Source: CAD feature listing. Evaluate the final solid. Frame: model axes, mm. Face numbers are marked on the shaded views. A direction names the side the tool comes from. Coordinates: 2 decimals unless noted, no trailing zeros. Write each loop counter-clockwise with the first axis right and the second up, starting at its lowest first coordinate (ties: lowest second). Pieces come first, ordered by that corner, then holes. Notation, with made-up numbers: (71, 26.25) -> (80, 26.25) arc R15 cw to (80, 41.25) -> close; hole circle Ø11 at (-2, 32.5). An arc over 180 degrees is marked (long way). One line per item, written item: value. Start each with the question number.
1. Section query A-A, the plane z = -31. Output: boundary loops of the cut face in (x, y), and give its area (3 significant figures).
2. Access query for the marked faces 4, 5, 6 and 7. Directions: +Z, -Z, +X, -X, +Y, -Y. A direction counts if a zero-diameter tool reaches every point of the face in a straight line with its end or side. Return the directions, or none.
3. Line query: line 1 (Y direction, x = -26, z = -4); line 2 (Z direction, x = -19.5, y = -22); line 3 (X direction, y = -29.5, z = -47). Output: solid intervals per line, ascending.
4. First-contact query: P1, Ø6, axis at x = 5, z = 36.5, coming from the +Y side; P2, Ø6, axis at x = 6, z = 11.5, coming from the -Y side; P3, Ø21.5, axis at y = 32.5, z = 18, coming from the -X side. Flat tips, straight axial feed; report the tip coordinate or a pass-through.
5. Mould query, pull axis Z, two halves, no side actions, for the marked faces 1, 2 and 3. Classes: released by +Z, released by -Z, zero draft, split by the parting line, or undercut.
from build123d import *

# Parameters (mm, degrees)
ENL_V_MAT_EXTRU_1_DEPTH      = 93.748315349
ENL_V_MAT_EXTRU_1_DEPTH_BACK = 93.748315349
ESQUISSE3_W                  = 49.590285902
ESQUISSE3_H                  = 55.327856271
ENL_V_MAT_EXTRU_2_DEPTH      = 93.748315349
ENL_V_MAT_EXTRU_2_DEPTH_BACK = 93.748315349


with BuildPart() as part:
    # Esquisse1 → Révolution1 (revolve)
    with BuildSketch(Plane(origin=(0, 0, 0), x_dir=(0, 0, -1), z_dir=(1, 0, 0)), mode=Mode.PRIVATE) as r_volution1_sk:
        with BuildLine():
            Line((-73.5, 0), (73.5, 0))
            Line((73.5, 0), (73.5, 25))
            Line((73.5, 25), (54.5, 25))
            ThreePointArc((54.5, 25), (53.085786438, 25.585786438), (52.5, 27))
            Line((52.5, 27), (52.5, 40))
            Line((52.5, 40), (21, 40))
            Line((21, 40), (18.5, 37.5))
            Line((18.5, 37.5), (-18.5, 37.5))
            Line((-18.5, 37.5), (-21, 40))
            Line((-21, 40), (-52.5, 40))
            Line((-52.5, 40), (-52.5, 27))
            ThreePointArc((-52.5, 27), (-53.085786438, 25.585786438), (-54.5, 25))
            Line((-54.5, 25), (-73.5, 25))
            Line((-73.5, 25), (-73.5, 0))
        make_face()
    revolve(r_volution1_sk.sketch.rotate(Axis((0, 0, 73.5), (0, 0, -1)), 90), axis=Axis((0, 0, 73.5), (0, 0, -1)))

    # Esquisse3 → Enlèv. mat.-Extru.1 (cut, two sides: drawn at the far end of the back side and taken through both)
    with BuildSketch(Plane.XY.offset(-ENL_V_MAT_EXTRU_1_DEPTH_BACK)):
        with Locations((-24.795142951, 27.663928136)):
            Rectangle(ESQUISSE3_W, ESQUISSE3_H)
    extrude(amount=ENL_V_MAT_EXTRU_1_DEPTH + ENL_V_MAT_EXTRU_1_DEPTH_BACK, mode=Mode.SUBTRACT)

    # Esquisse4 → Enlèv. mat.-Extru.2 (cut, two sides: drawn at the far end of the back side and taken through both)
    with BuildSketch(Plane.XY.offset(-ENL_V_MAT_EXTRU_2_DEPTH_BACK)):
        with BuildLine():
            Line((0, 7), (12, 7))
            ThreePointArc((12, 7), (15, 10), (12, 13))
            Line((12, 13), (0, 13))
            Line((0, 13), (0, 7))
        make_face()
    extrude(amount=ENL_V_MAT_EXTRU_2_DEPTH + ENL_V_MAT_EXTRU_2_DEPTH_BACK, mode=Mode.SUBTRACT)


solid = part.part
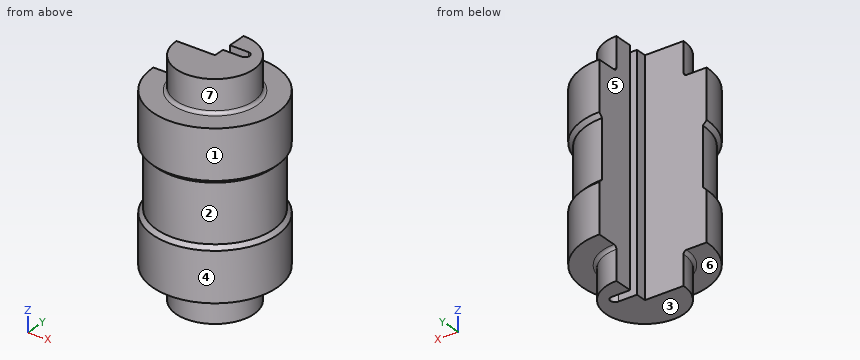
Computed values:
1. outline: (-40, 0) arc R40 ccw (long way) to (0, 40) -> (0, 13) -> (12, 13) arc R3 cw to (12, 7) -> (0, 7) -> (0, 0) -> close
1. area: 3,680 mm²
2. face 4: +Z, -Z
2. face 5: +Z, -Z, -X, +Y
2. face 6: -Z
2. face 7: +Z
3. line 1: y = -27.02 to 0
3. line 2: z = -52.5 to 52.5
3. line 3: x = -27.01 to 27.01
4. P1: stops at y = 39.95
4. P2: stops at y = -37.38
4. P3: stops at x = 0
5. face 1: zero draft
5. face 2: undercut
5. face 3: released by -Z
